Geometry check sheet. Reference: the model listing, model coordinates, mm. Give positions to 0.01 mm unless a question says otherwise; leave off trailing zeros. Write each loop counter-clockwise with the first axis right and the second up, starting at its lowest first coordinate (ties: lowest second). Pieces come first, ordered by that corner, then holes. Notation, with made-up numbers: (47, -13) -> (95, -13) arc R29 cw to (95, 15) -> close; hole circle Ø7 at (66, 39.5). An arc over 180 degrees is marked (long way). Write item = value, one per line. Start each with the question number.
1. Cross-section at C-C, the plane y = 234. Record the cut outline in (x, z).
2. Cross-section at A-A, the plane y = 124.5. Record the cut outline in (x, z).
3. Thickness scan on line 1 along Y through (x, z) = (11, 14.75); line 2 along X through (y, z) = (110, 16.55); line 3 along X through (y, z) = (153, 15.05). Record the ranges inside material, lowest first.
4. Mould release check, pull along X, two halves, no side actions. Record for faces 1 (the cylindrical face through (1.04, 5.713, 15.479)), 2 (the cylindrical face through (0.69, 142.623, 15.479)), 3 (the flat face through (3, 130, 17)): pulls with the +X half, pulls with the -X half, needs draft (parallel to the pull), parting line crosses it, or undercut.
5. Cross-section at B-B, the plane z = 15.5. State how many separate pieces and enclosed holes the cut face has, plus the area to 3 significant figures.
6. Depth check by flat-ended pin: P1, Ø2.5, axis at x = -16.51, y = 60.71, coming from the -Z side; P2, Ø0.9, axis at x = 25, z = 16, coming from the +Y side; P3, Ø1.5, axis at x = 9.5, z = 16, coming from the +Y side. Enter the tip coordinate at first touch or a pass-through.
Autodesk Inventor part; units mm, degrees
ref_plane "YZ Plane" through (0, 0, 0) normal (1, 0, 0) x (0, 1, 0)
ref_plane "XZ Plane" through (0, 0, 0) normal (0, 1, 0) x (-1, 0, 0)
ref_plane "XY Plane" through (0, 0, 0) normal (0, 0, 1) x (1, 0, 0)
ref_plane "Work Plane2" through (0.4904, 0, 14) normal (0, 0, 1) x (1, 0, 0)
sketch "Sketch1" plane through (0.4904, 0, 14) normal (0, 0, 1) x (1, 0, 0)
  line L0 (-25, 225.7065) -> (25, 225.7065)
  line L1 (25, 225.7065) -> (25, 5.7065)
  line L2 (25, 5.7065) -> (-25, 5.7065)
  line L3 (-25, 5.7065) -> (-25, 225.7065)
  line L4 (-25, 225.7065) -> (25, 225.7065)
  line L5 (20, 5.7065) -> (-20, 5.7065)
  circle A0 centre (0, 30.7065) radius 3.5
  circle A1 centre (0, 30.7065) radius 25
  circle A2 centre (0, 225.7065) radius 25
  line L6 (-25, 30.7065) -> (-25, 225.7065)
  line L7 (25, 225.7065) -> (25, 30.7065)
  point P0 (-0.4904, 0)
  dimension "d19" = 50
  dimension "d6" = 220
  dimension "d7" = 0
  dimension "d9" = 50
  dimension "d10" = 25
  dimension "d11" = 25
  dimension "d12" = 25
  dimension "d13" = 0
extrude "Extrusion1" add sketch "Sketch1" along normal blind 3 contours A2 L0 | A2 L1 A1 L3 | L0 A2 | A1
sketch "Sketch2" plane through (0.4904, 0, 17) normal (0, 0, 1) x (1, 0, 0)
  arc A0 (25, 225.7065) -> (-25, 225.7065) centre (0, 225.7065) ccw
  circle A1 centre (0, 225.7065) radius 5
  point P0 (-0.4904, 0)
  dimension "d16" = 10
extrude "Extrusion2" cut sketch "Sketch2" against normal blind 3
sketch "Sketch4" plane through (0.4904, 0, 17) normal (0, 0, 1) x (1, 0, 0)
  arc A0 (20.4946, 25.2317) -> (20.5054, 36.1404) centre (18, 30.6886) ccw
  line L0 (20.5054, 36.1404) -> (10.4453, 40.7636)
  arc A1 (10.4252, 20.6286) -> (10.4453, 40.7636) centre (0, 30.7065) ccw
  line L1 (10.4252, 20.6286) -> (20.4946, 25.2317)
  circle A2 centre (18, 30.6886) radius 2.5
  arc A3 (-20.5376, 36.019) -> (-20.4622, 25.1105) centre (-18, 30.582) ccw
  line L2 (-20.4622, 25.1105) -> (-11.0226, 20.8627)
  arc A4 (-11.1577, 40.3969) -> (-11.0226, 20.8627) centre (0, 30.7065) ccw
  line L3 (-11.1577, 40.3969) -> (-20.5376, 36.019)
  circle A5 centre (-18, 30.582) radius 2.5
  point P0 (-0.4904, 0)
extrude "Extrusion4" cut sketch "Sketch4" against normal blind 10 contours A2 | A5
sketch "Sketch6" plane through (0.4904, 0, 14) normal (0, 0, -1) x (-1, 0, 0)
  circle A0 centre (0, 42.7065) radius 2
  circle A1 centre (-12, 30.7065) radius 2
  circle A2 centre (0, 18.7065) radius 2
  circle A3 centre (12, 30.7065) radius 2
  point P0 (0.4904, 0)
extrude "Extrusion6" cut sketch "Sketch6" against normal blind 10
sketch "Sketch7" plane through (0.4904, 0, 14) normal (0, 0, -1) x (-1, 0, 0)
  circle A0 centre (-12, 30.7065) radius 2
  circle A1 centre (0, 18.7065) radius 2
  circle A2 centre (12, 30.7065) radius 2
  circle A3 centre (0, 42.7065) radius 2
  circle A4 centre (-18, 30.6886) radius 2.5
  circle A5 centre (18, 30.582) radius 2.5
  circle A6 centre (0, 225.7065) radius 5
  line L0 (25, 225.7065) -> (25, 30.7065)
  line L1 (-25, 30.7065) -> (-25, 225.7065)
  arc A7 (-25, 30.7065) -> (25, 30.7065) centre (0, 30.7065) ccw
  circle A8 centre (0, 30.7065) radius 3.5
  circle A9 centre (0.668, 146.5279) radius 12.5
  circle A10 centre (9.168, 146.5279) radius 2.3813
  circle A11 centre (-7.832, 146.5279) radius 2.3813
  circle A12 centre (0.668, 155.0279) radius 1.5
  circle A13 centre (0.668, 138.0279) radius 1.5
  circle A14 centre (0.668, 146.5279) radius 4
  arc A15 (25, 225.7065) -> (-25, 225.7065) centre (0, 225.7065) ccw
  point P0 (0.4904, 0)
  dimension "d60" = 8
extrude "Extrusion7" cut sketch "Sketch7" against normal blind 10 contours A12 | A13 | A14
sketch "Sketch10" plane through (0.4904, 0, 17) normal (0, 0, 1) x (1, 0, 0)
  line L0 (17, 181.6543) -> (2, 181.6543)
  line L1 (2, 181.6543) -> (2, 176.6543)
  line L2 (2, 176.6543) -> (17, 176.6543)
  line L3 (17, 176.6543) -> (17, 181.6543)
  line L4 (25, 30.7065) -> (25, 225.7065)
  point P0 (-0.4904, 0)
  dimension "d67" = 15
  dimension "d68" = 5
  dimension "d69" = 8
extrude "Extrusion10" cut sketch "Sketch10" against normal blind 10
fillet "Fillet1" radius 2 4 edges at (17.4904, 176.6543, 15.5) (17.4904, 181.6543, 15.5) (2.4904, 181.6543, 15.5) (2.4904, 176.6543, 15.5)
sketch "Sketch11" plane through (0.4904, 0, 17) normal (0, 0, 1) x (1, 0, 0)
  arc A0 (20.5376, 220.3941) -> (20.4622, 231.3026) centre (18, 225.831) ccw
  line L0 (20.4622, 231.3026) -> (11.0226, 235.5503)
  arc A1 (11.1577, 216.0162) -> (11.0226, 235.5503) centre (0, 225.7065) ccw
  line L1 (11.1577, 216.0162) -> (20.5376, 220.3941)
  circle A2 centre (18, 225.831) radius 2.5
  arc A3 (-20.4946, 231.1813) -> (-20.5054, 220.2726) centre (-18, 225.7245) ccw
  line L2 (-20.5054, 220.2726) -> (-10.4453, 215.6494)
  arc A4 (-10.4252, 235.7844) -> (-10.4453, 215.6494) centre (0, 225.7065) ccw
  line L3 (-10.4252, 235.7844) -> (-20.4946, 231.1813)
  circle A5 centre (-18, 225.7245) radius 2.5
  circle A6 centre (3.5, 208.0565) radius 1.5
  circle A7 centre (3.5, 197.2565) radius 1.5
  line L4 (15, 176.6543) -> (4, 176.6543)
  arc A8 (2, 178.6543) -> (4, 176.6543) centre (4, 178.6543) ccw
  line L5 (2, 178.6543) -> (2, 179.6543)
  arc A9 (4, 181.6543) -> (2, 179.6543) centre (4, 179.6543) ccw
  line L6 (4, 181.6543) -> (15, 181.6543)
  arc A10 (17, 179.6543) -> (15, 181.6543) centre (15, 179.6543) ccw
  line L7 (17, 179.6543) -> (17, 178.6543)
  arc A11 (15, 176.6543) -> (17, 178.6543) centre (15, 178.6543) ccw
  circle A12 centre (-0.668, 146.5279) radius 4
  circle A13 centre (-0.668, 138.0279) radius 1.5
  circle A14 centre (-0.668, 155.0279) radius 1.5
  circle A15 centre (12, 30.7065) radius 2
  circle A16 centre (0, 18.7065) radius 2
  circle A17 centre (-12, 30.7065) radius 2
  circle A18 centre (0, 42.7065) radius 2
  circle A19 centre (18, 30.6886) radius 2.5
  circle A20 centre (-18, 30.582) radius 2.5
  circle A21 centre (0, 225.7065) radius 5
  line L8 (-25, 225.7065) -> (-25, 30.7065)
  arc A22 (-25, 30.7065) -> (25, 30.7065) centre (0, 30.7065) ccw
  line L9 (25, 30.7065) -> (25, 225.7065)
  arc A23 (25, 225.7065) -> (-25, 225.7065) centre (0, 225.7065) ccw
  circle A24 centre (0, 30.7065) radius 3.5
  circle A25 centre (18.3, 208.0565) radius 1.5
  point P0 (-0.4904, 0)
extrude "Extrusion11" cut sketch "Sketch11" against normal blind 10 contours A2 | A5
sketch "Sketch12" plane through (0.4904, 0, 17) normal (0, 0, 1) x (1, 0, 0)
  circle A0 centre (17, 60.7065) radius 1.5
  circle A1 centre (-17, 60.7065) radius 1.5
  circle A2 centre (-17, 110.7065) radius 1.5
  circle A3 centre (17, 110.7065) radius 1.5
  circle A4 centre (-17, 160.7065) radius 1.5
  line L0 (-25, 225.7065) -> (-25, 30.7065)
  line L1 (25, 30.7065) -> (25, 225.7065)
  circle A5 centre (0, 30.7065) radius 3.5
  circle A6 centre (17, 160.7065) radius 1.5
  point P0 (-0.4904, 0)
  dimension "d75" = 3
  dimension "d76" = 3
  dimension "d77" = 3
  dimension "d78" = 3
  dimension "d79" = 3
  dimension "d80" = 8
  dimension "d81" = 8
  dimension "d82" = 8
  dimension "d83" = 8
  dimension "d84" = 8
  dimension "d85" = 30
  dimension "d86" = 30
  dimension "d87" = 50
  dimension "d88" = 50
  dimension "d89" = 50
  dimension "d90" = 3
  dimension "d91" = 8
  dimension "d92" = 50
extrude "Extrusion12" cut sketch "Sketch12" against normal blind 10 contours A0 | A1 | A2 | A3 | A4 | A6
sketch "Sketch13" plane through (0.4904, 0, 17) normal (0, 0, 1) x (1, 0, 0)
  line L0 (15.5, 214.3827) -> (30.5, 214.3827)
  line L1 (30.5, 214.3827) -> (30.5, 249.3827)
  line L2 (30.5, 249.3827) -> (15.5, 249.3827)
  line L3 (15.5, 249.3827) -> (15.5, 214.3827)
  circle A0 centre (18, 225.831) radius 2.5
  point P0 (-0.4904, 0)
  point P1 (15.5, 225.831)
  dimension "d95" = 15
  dimension "d96" = 35
extrude "Extrusion13" add sketch "Sketch13" against normal blind 3
sketch "Sketch14" plane through (0.4904, 0, 14) normal (0, 0, -1) x (-1, 0, 0)
  circle A0 centre (-18.15, 246.2827) radius 1.5
  circle A1 centre (-18.15, 212.3827) radius 1.5
  circle A2 centre (-28.95, 212.3827) radius 1.5
  point P0 (0.4904, 0)
extrude "Extrusion14" cut sketch "Sketch14" against normal blind 3 contours A0 | A1
fillet "Fillet2" radius 3 5 edges at (15.9904, 245.3216, 15.5) (15.9904, 249.3827, 15.5) (30.9904, 249.3827, 15.5) (30.9904, 214.3827, 15.5) (25.4904, 214.3827, 15.5)
properties part number "Link2Base"
Answers:
q1.outline = (-23.09, 14) -> (30.99, 14) -> (30.99, 17) -> (-23.09, 17) -> close
q2.outline = (-24.51, 14) -> (25.49, 14) -> (25.49, 17) -> (-24.51, 17) -> close
q3.line_1 = 8.02 to 29.37, 32.04 to 176.65, 181.65 to 248.39
q3.line_2 = -24.51 to -17.83, -15.19 to 16.17, 18.81 to 25.49
q3.line_3 = -24.51 to 25.49
q4.face_1 = parting line crosses it
q4.face_2 = undercut
q4.face_3 = needs draft
q5.separate_pieces = 1
q5.enclosed_holes = 22
q5.area = 11,600 mm^2
q6.P1 = through
q6.P2 = 249.38
q6.P3 = 249.3
